Read the model definition and answer for the solid it produces. Units are mm, in the model's axes. Face numbers are marked on the shaded views. Coordinates: 2 decimals unless noted, no trailing zeros. Write each loop counter-clockwise with the first axis right and the second up, starting at its lowest first coordinate (ties: lowest second). Pieces come first, ordered by that corner, then holes. Notation, with made-up numbers: (51.5, -22.5) -> (66.5, -22.5) arc R10 cw to (66.5, -4.5) -> close; hole circle Ø8 at (3, 69). An arc over 180 degrees is marked (long way). Return JSON: item names as keys, results as strings.
Autodesk Inventor part; units mm, degrees
ref_plane "YZ Plane" through (0, 0, 0) normal (1, 0, 0) x (0, 1, 0)
ref_plane "XZ Plane" through (0, 0, 0) normal (0, 1, 0) x (-1, 0, 0)
ref_plane "XY Plane" through (0, 0, 0) normal (0, 0, 1) x (1, 0, 0)
sketch "Sketch1" plane through (0, 0, 0) normal (0, 1, 0) x (-1, 0, 0)
  line L0 (193.5, 0) -> (235, 0)
  line L1 (235, 0) -> (235, 2)
  line L2 (235, 2) -> (300, 2)
  line L3 (300, 2) -> (300, 37)
  line L4 (300, 37) -> (193.5, 37)
  line L5 (193.5, 37) -> (193.5, 0)
  line L6 (0, 0) -> (0, 37)
  line L7 (0, 37) -> (193.5, 37) construction
  line L8 (0, 0) -> (193.5, 0) construction
  line L9 (-610, 610) -> (-573, 610) construction
  line L10 (-573, 610) -> (-573, 803.5) construction
  line L11 (-573, 803.5) -> (-610, 803.5)
  line L12 (-610, 803.5) -> (-610, 610) construction
  line L13 (-573, 803.5) -> (-573, 910)
  line L14 (-573, 910) -> (-608, 910)
  line L15 (-608, 910) -> (-608, 845)
  line L16 (-608, 845) -> (-610, 845)
  line L17 (-610, 845) -> (-610, 803.5)
  dimension "d0" = 387
  dimension "d1" = 600
  dimension "d2" = 470
  dimension "d3" = 2
  dimension "d4" = 37
  dimension "d6" = 2
  dimension "d7" = 37
  dimension "d8" = 387
  dimension "d9" = 470
  dimension "d10" = 600
  dimension "d11" = 610
  dimension "d12" = 610
revolve "Revolution1" add sketch "Sketch1" angle 360 about axis through (0, 0, 0) along (0, 0, 1) contours L5 L4 L3 L2 L1 L0
revolve "Revolution2" add sketch "Sketch1" angle 360 about axis through (610, 0, 610) along (-1, 0, 0) contours L11 L17 L16 L15 L14 L13
sketch "Sketch2" plane through (0, 0, 0) normal (0, 1, 0) x (-1, 0, 0)
  line L0 (-573, 803.5) -> (-573, 910)
  line L1 (300, 37) -> (193.5, 37)
  line L2 (0, 0) -> (0, 37)
  line L3 (-610, 610) -> (-573, 610)
  arc A0 (0, 37) -> (-573, 610) centre (-573, 37) ccw
sketch "Sketch3" plane through (0, 0, 37) normal (0, 0, 1) x (1, 0, 0)
  circle A0 centre (0, 0) radius 193.5
  circle A1 centre (0, 0) radius 193.5
  circle A2 centre (0, 0) radius 204.6
  dimension "d14" = 409.2
sweep "Sweep1" add profiles "Sketch3" path "Sketch2" path curves L2 A0 L3
sketch "Sketch6" plane through (0, 0, 2) normal (0, 0, -1) x (-1, 0, 0)
  circle A0 centre (0, 0) radius 300
  circle A1 centre (-52.6744, -264.812) radius 14.75
  circle A2 centre (0, 0) radius 270 construction
  line L0 (-52.6744, -264.812) -> (0, 0) construction
  line L1 (0, 0) -> (0, -270) construction
  dimension "d20" = 11.25
  dimension "d21" = 29.5
  dimension "d22" = 540
extrude "Extrusion1" cut sketch "Sketch6" against normal up to surface (35 mm away) contours A1
pattern_circular "Circular Pattern1" count 16 over 360 about axis through (0, 0, 19.5) along (0, 0, -1) of "Extrusion1"
sketch "Sketch7" plane through (608, 0, 610) normal (1, 0, 0) x (0, 0, -1)
  circle A0 centre (0, 0) radius 235
  circle A1 centre (-52.6744, -264.812) radius 14.75
  circle A2 centre (0, 0) radius 270 construction
  line L0 (-52.6744, -264.812) -> (0, 0) construction
  line L1 (0, 0) -> (0, -270) construction
  dimension "d25" = 11.25
  dimension "d26" = 29.5
  dimension "d27" = 540
extrude "Extrusion2" cut sketch "Sketch7" against normal up to surface (35 mm away) contours A1
pattern_circular "Circular Pattern2" count 16 over 360 about axis through (590.5, 0, 610) along (-1, 0, 0) of "Extrusion2"
equation "\"d0\" = d"
equation "\"d1\" = D1"
equation "\"d2\" = D2"
equation "\"d4\" = C1"
equation "\"d7\" = C1"
equation "\"d8\" = d"
equation "\"d9\" = D2"
equation "\"d10\" = D1"
equation "\"d11\" = BB"
equation "\"d12\" = BB"
equation "\"d14\" = d + 2 * t"
equation "\"d21\" = L"
equation "\"d22\" = K1"
equation "\"d26\" = L"
equation "\"d27\" = K1"
equation "\"D1\" = 600"
equation "\"C1\" = 37"
equation "\"t\" = 11.1"
equation "\"d\" = 387"
equation "\"BB\" = 610"
equation "\"D2\" = 470"
equation "\"K1\" = 540"
equation "\"L\" = 29.5"
properties part number "GB/T 17185 400-PN20 \"F90E(L) RF\"" material "Steel"
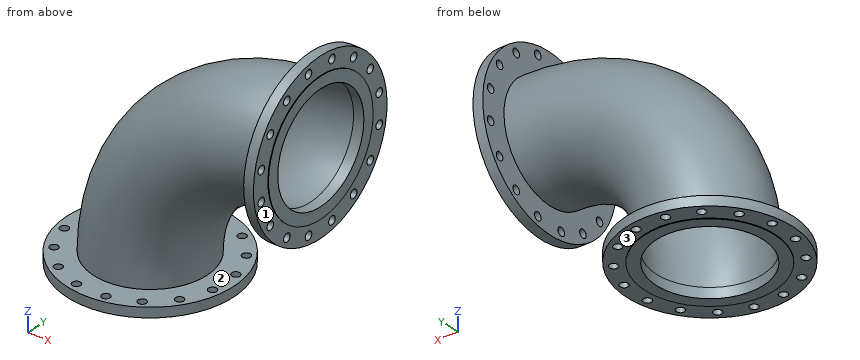
1. Consider L1, parallel to X at y = 94, z = 391; L2, parallel to Z at x = -7, y = -273; L3, parallel to X at y = 93, z = 276.5. Determine where each line is inside the solid, lowest interval first.
Taken from the geometry:
{"L1": "x = -93.56 to -79.26, 378.6 to 406.33, 573 to 608", "L2": "z = 2 to 37", "L3": "x = -143.26 to -130.01, 248.5 to 264.24"}
2. For a pull along Z with two mould halves and no side action, classify the marked faces 1, 2 and 3 as +Z half, -Z half, draft (parallel to the pull), parting line (faces both ways), or undercut.
Taken from the geometry:
{"face 1": "draft", "face 2": "undercut", "face 3": "-Z half"}
3. The part is cut by section B-B (x = -50). Count the separate pieces of the cut face and the enclosed holes in it, then the cut area to 3 significant figures.
Taken from the geometry:
{"separate pieces": "3", "enclosed holes": "0", "area": "20,600 mm2"}
4. Flat-ended cylindrical pins translate along their axes: pin 1 Ø17.5 at (x, y) = (-52.67, 264.81) entering from +Z; pin 2 Ø4 at (x, y) = (-16, 238.5) entering from +Z; pin 3 Ø10 at (x, y) = (480, 12) entering from -Z; pin 4 Ø4 at (x, y) = (-97.5, 7.5) entering from +Z. Find the tip coordinate at first contact, or state that the pin passes through.
Taken from the geometry:
{"pin 1": "passes through", "pin 2": "stops at z = 37", "pin 3": "stops at z = 392.46", "pin 4": "stops at z = 433.94"}
5. The part is cut by section A-A (y = 0). Determine the outline of the cut face in (x, z), then the cut area to 3 significant figures.
Taken from the geometry:
{"outline": "(-300, 2) -> (-235, 2) -> (-235, 0) -> (-193.5, 0) -> (-193.5, 37) arc R766.5 cw to (573, 803.5) -> (610, 803.5) -> (610, 845) -> (608, 845) -> (608, 910) -> (573, 910) -> (573, 814.6) arc R777.6 ccw to (-204.6, 37) -> (-300, 37) -> close; (193.5, 0) -> (235, 0) -> (235, 2) -> (300, 2) -> (300, 37) -> (204.6, 37) arc R368.4 cw to (573, 405.4) -> (573, 310) -> (608, 310) -> (608, 375) -> (610, 375) -> (610, 416.5) -> (573, 416.5) arc R379.5 ccw to (193.5, 37) -> close", "area": "35,200 mm2"}
6. The part is cut by section C-C (y = -81.5). Determine the outline of the cut face in (x, z), then the cut area to 3 significant figures.
Taken from the geometry:
{"outline": "(-288.72, 2) -> (-220.41, 2) -> (-220.41, 0) -> (-175.5, 0) -> (-175.5, 37) arc R748.5 cw to (573, 785.5) -> (610, 785.5) -> (610, 830.41) -> (608, 830.41) -> (608, 898.72) -> (573, 898.72) -> (573, 797.67) arc R760.67 ccw to (-187.67, 37) -> (-288.72, 37) -> close; (175.5, 0) -> (220.41, 0) -> (220.41, 2) -> (288.72, 2) -> (288.72, 37) -> (187.67, 37) arc R385.33 cw to (573, 422.33) -> (573, 321.28) -> (608, 321.28) -> (608, 389.59) -> (610, 389.59) -> (610, 434.5) -> (573, 434.5) arc R397.5 ccw to (175.5, 37) -> close", "area": "38,100 mm2"}
